Part model, mm, in its own coordinate system. A direction names the side the tool comes from. Coordinates: 2 decimals unless noted, no trailing zeros. Loops run counter-clockwise (first coordinate to the right, second up) from the corner with the lowest first, then second, coordinate; pieces in that order, holes last. Notation, with made-up numbers: (-28.75, 50.25) - (-18.75, 50.25) arc R22 cw to (-18.75, 66.25) - close; hole circle Ø5 at (3.5, 87). An arc over 180 degrees is marked (long way). One line per question, with ' | ' between items. Start each with the question number.
from build123d import *

# Parameters (mm, degrees)
SKETCH_1_R          = 1.6
SKETCH_1_R_2        = 1.15
SKETCH_1_W          = 36
SKETCH_1_H          = 14
EXTRUDE_1_DEPTH     = 2
CUT_EXTRUDE_1_DEPTH = 121.516596367
FILLET_1_R          = 2
FILLET_2_R          = 1
FILLET_3_R          = 1


with BuildPart() as part:
    # 草图1 → 凸台-拉伸1 (new body)
    with BuildSketch(Plane.XY):
        Polygon((0, 0), (0, 60), (75, 60), (104.5, 42), (104.5, 10), (91.5, 10), (91.5, 0), (73.5, 0), (73.5, 6), (60.5, 6), (60.5, 0), (33, 0), (33, 6), (20, 6), (20, 0), align=None)
        with Locations((86.5, 5)):
            Circle(SKETCH_1_R, mode=Mode.SUBTRACT)
        with Locations((5, 5)):
            Circle(SKETCH_1_R, mode=Mode.SUBTRACT)
        with Locations((60.6, 48.1)):
            Circle(SKETCH_1_R_2, mode=Mode.SUBTRACT)
        with Locations((60.6, 30.1)):
            Circle(SKETCH_1_R_2, mode=Mode.SUBTRACT)
        with Locations((15.4, 48.1)):
            Circle(SKETCH_1_R_2, mode=Mode.SUBTRACT)
        with Locations((15.4, 30.1)):
            Circle(SKETCH_1_R_2, mode=Mode.SUBTRACT)
        with Locations((87.5, 46.515606374)):
            Circle(SKETCH_1_R, mode=Mode.SUBTRACT)
        with Locations((55, 57)):
            Circle(SKETCH_1_R, mode=Mode.SUBTRACT)
        with Locations((35, 57)):
            Circle(SKETCH_1_R, mode=Mode.SUBTRACT)
        with Locations((5, 55)):
            Circle(SKETCH_1_R, mode=Mode.SUBTRACT)
        with BuildLine():
            Line((71.5, 12), (16, 12))
            ThreePointArc((16, 12), (12, 16), (16, 20))
            Line((16, 20), (71.5, 20))
            ThreePointArc((71.5, 20), (75.5, 16), (71.5, 12))
        make_face(mode=Mode.SUBTRACT)
        with Locations((38, 39.1)):
            Rectangle(SKETCH_1_W, SKETCH_1_H, mode=Mode.SUBTRACT)
    extrude(amount=EXTRUDE_1_DEPTH)

    # 草图2 → 切除-拉伸1 (cut, through all)
    with BuildSketch(Plane(origin=(0, 0, 0), x_dir=(-1, 0, 0), z_dir=(0, 0, -1))):
        with BuildLine():
            Line((-87.5, 37), (-87.5, 18))
            ThreePointArc((-87.5, 18), (-92.5, 13), (-97.5, 18))
            Line((-97.5, 18), (-97.5, 37))
            ThreePointArc((-97.5, 37), (-92.5, 42), (-87.5, 37))
        make_face()
        with BuildLine():
            Line((-71.5, 50), (-71.5, 29))
            ThreePointArc((-71.5, 29), (-75.5, 25), (-79.5, 29))
            Line((-79.5, 29), (-79.5, 50))
            ThreePointArc((-79.5, 50), (-75.5, 54), (-71.5, 50))
        make_face()
    extrude(amount=-CUT_EXTRUDE_1_DEPTH, mode=Mode.SUBTRACT)

    # 圆角1
    fillet_1_edges = [part.edges().sort_by_distance(p)[0] for p in [
        (0, 0, 1),
        (0, 60, 1),
        (75, 60, 1),
        (104.5, 42, 1),
        (104.5, 10, 1),
        (91.5, 10, 1),
        (91.5, 0, 1),
        (73.5, 0, 1),
        (60.5, 0, 1),
        (33, 0, 1),
        (20, 0, 1),
    ]]
    fillet(fillet_1_edges, radius=FILLET_1_R)

    # 圆角2
    fillet_2_edges = [part.edges().sort_by_distance(p)[0] for p in [
        (56, 32.1, 1),
        (56, 46.1, 1),
        (20, 46.1, 1),
        (20, 32.1, 1),
    ]]
    fillet(fillet_2_edges, radius=FILLET_2_R)

    # 圆角3
    fillet_3_edges = [part.edges().sort_by_distance(p)[0] for p in [
        (73.5, 6, 1),
        (60.5, 6, 1),
        (33, 6, 1),
        (20, 6, 1),
    ]]
    fillet(fillet_3_edges, radius=FILLET_3_R)


solid = part.part
1) Mould opens along Y. For faces 4 (the flat face through (38, 60, 1)), 5 (the flat face through (47, 0, 1)), 6 (the flat face through (20, 4, 1)), 7 (the cylindrical face through (92.6, 42, 1)) say: +Y half, -Y half, draft (parallel to the pull), parting line (faces both ways), or undercut.
2) Tool access for faces 1 (the cylindrical face through (92.4, 13, 1)), 2 (the flat face through (33, 3, 1)), 3 (the flat face through (53, 30, 2)): list every direction of +Z, -Z, +X, -X, +Y, -Y with a clear straight run to the whole face (end or side of a thin tool).
3) Band-saw the part on A-A on y = 16. List the corners of the cut face in (x, z).
4) Band-saw the part on B-B on z = 1.3. Count the separate pieces of the cut face and the enclosed holes in it, then the cut area to 3 significant figures.
5) Pin check, flat tips, straight feed: pin 1 Ø1.9 at (x, y) = (55, 57) entering from -Z; pin 2 Ø2 at (x, y) = (88.5, 42.5) entering from -Z; pin 3 Ø1 at (y, z) = (5.5, 1) entering from +X. Stop position of each tip, or through.
6) Wall check: line 1 along X through (y, z) = (30, 1.75); line 2 along Y through (x, z) = (23, 0.45); line 3 along Y through (x, z) = (55, 0.55). Give the ranges that are in metal, low to high. Write a range as [from, to].
Values found:
1) face 4: +Y half | face 5: -Y half | face 6: draft | face 7: undercut
2) face 1: +Z, -Z | face 2: +Z, -Z, -Y | face 3: +Z, +X, -X, +Y, -Y
3) outline: (0, 0) - (12, 0) - (12, 2) - (0, 2) - close; (75.5, 0) - (87.92, 0) - (87.92, 2) - (75.5, 2) - close; (97.08, 0) - (104.5, 0) - (104.5, 2) - (97.08, 2) - close
4) separate pieces: 1 | enclosed holes: 14 | area: 4,160 mm²
5) pin 1: through | pin 2: z = 0 | pin 3: x = 91.5
6) line 1: [0, 14.25], [16.55, 59.45], [61.75, 71.5], [79.5, 87.5], [97.5, 104.5] | line 2: [6, 12], [20, 32.1], [46.1, 60] | line 3: [0, 12], [20, 32.1], [46.1, 55.4], [58.6, 60]
